Work out the finished part from the listing and answer in its coordinate system (mm). A direction names the side the tool comes from. Round coordinates to 2 decimals unless told otherwise and drop trailing zeros. Order: outer loops, then holes, each group sorted by start corner. A loop starts at its lowest first (then second) coordinate and runs counter-clockwise, first axis right, second up.
from build123d import *

# Parameters (mm, degrees)
REVOLVE2_ANGLE      = 10
SKETCH2_R           = 10
BOSS_EXTRUDE1_DEPTH = 10


with BuildPart() as part:
    # Sketch1 → Revolve2 (revolve)
    with BuildSketch(Plane(origin=(0, 0, 0), x_dir=(1, 0, 0), z_dir=(0, 1, 0))):
        with BuildLine():
            Line((40, 1.5), (41.5, 1.5))
            ThreePointArc((41.5, 1.5), (40, 0), (41.5, -1.5))
            Line((41.5, -1.5), (40, -1.5))
            Line((40, -1.5), (0, -1.5))
            Line((0, -1.5), (0, 1.5))
            Line((0, 1.5), (40, 1.5))
        make_face()
    revolve(axis=Axis((0, 0, -1.5), (0, 0, 1)), revolution_arc=REVOLVE2_ANGLE)

    # Sketch2 → Boss-Extrude1 (add)
    with BuildSketch(Plane.XY.offset(1.5)):
        Circle(SKETCH2_R)
    extrude(amount=BOSS_EXTRUDE1_DEPTH)


solid = part.part
Item 1: Find section D-D (z = 0.75). Write down the section's boundary in (x, y), plus the area to 3 significant figures.
Item 2: Find section B-B (x = 0.5). Write down the section's boundary in (y, z).
Item 3: Given pin 1 (1.5 mm diameter, centred on x = 5.5, z = 4, fed in from -Y); pin 2 (3.5 mm diameter, centred on x = 27.5, y = 4, fed in from +Z); pin 3 (3.5 mm diameter, centred on x = 23.5, z = 0.5, fed in from -Y), each flat-ended and moving along its own axis, determine where each tip first touches the part or whether it passes through.
Item 4: For a pull along Y with two mould halves and no side action, classify faces 3 (the face through (29, 3, 1.5)), 4 (the face through (-2.17, -9.76, 6.43)), 5 (the face through (20.721, 3.654, -0.021)) as released by +Y, released by -Y, zero draft, split by the parting line, or undercut.
Item 5: Find section A-A (z = 4.75). Write down the section's boundary in (x, y), plus the area to 3 significant figures.
Item 6: Find section C-C (y = -4). Write down the section's boundary in (x, z), plus the area to 3 significant figures.
Item 7: A tool of negligible diameter and unlimited length cuts with its end or side. For faces 1 (the face through (26, 3, -1.5)), 2 (the face through (21, 0, 0)), from which of +Z, -Z, +X, -X, +Y, -Y can it reach the whole face along a straight path? Write none if from no direction.
Item 8: Find the intervals of material crossed by line 1 along Z through (x, y) = (-2.5, -8.25); line 2 along Z through (x, y) = (10, 1); line 3 along X through (y, z) = (-0.25, 4.5), in increasing order.
Model answer:
1. outline: (0, 0) - (40.2, 0) arc R40.2 ccw to (39.59, 6.98) - close
1. area: 141 mm2
2. outline: (-9.99, 1.5) - (0, 1.5) - (0, -1.5) - (0.09, -1.5) - (0.09, 1.5) - (9.99, 1.5) - (9.99, 11.5) - (-9.99, 11.5) - close
3. pin 1: stops at y = -8.8
3. pin 2: stops at z = 1.5
3. pin 3: stops at y = 0
4. face 3: zero draft
4. face 4: split by the parting line
4. face 5: released by +Y
5. outline: circle Ø20 at (0, 0)
5. area: 314 mm2
6. outline: (-9.17, 1.5) - (9.17, 1.5) - (9.17, 11.5) - (-9.17, 11.5) - close
6. area: 183 mm2
7. face 1: -Z, +X, -X, +Y, -Y
7. face 2: -Z, +X, -X, -Y
8. line 1: z = 1.5 to 11.5
8. line 2: z = -1.5 to 1.5
8. line 3: x = -10 to 10
